The listing builds one solid part. Answer for the finished solid, in the listing's coordinates (mm). A direction names the side the tool comes from. Coordinates: 2 decimals unless noted, no trailing zeros. Order: outer loops, then holes, each group sorted by start corner. A loop starts at its lowest first (then second) coordinate and runs counter-clockwise, first axis right, second up. Notation, with made-up numbers: (-9.5, 78) -> (22.5, 78) arc R24 cw to (22.5, 112) -> close; hole circle Ø11 at (-24.75, 79). An arc over 180 degrees is marked (long way). Return JSON: item names as keys, results as strings.
from build123d import *

# Parameters (mm, degrees)
EXTRUDE_1_DEPTH     = 7
SKETCH_2_R          = 2
CUT_EXTRUDE_1_DEPTH = 10
SKETCH_3_W          = 40
SKETCH_3_H          = 40
CUT_EXTRUDE_2_DEPTH = 7
FILLET_1_R          = 2
FILLET_2_R          = 2
SKETCH_4_R          = 2
CUT_EXTRUDE_3_DEPTH = 90


with BuildPart() as part:
    # 草图1 → 凸台-拉伸1 (new body)
    with BuildSketch(Plane.XY):
        Polygon((0, 0), (220, 0), (224.357787137, -49.809734905), (-4.357787137, -49.809734905), align=None)
    extrude(amount=EXTRUDE_1_DEPTH)

    # 草图2 → 切除-拉伸1 (cut)
    with BuildSketch(Plane(origin=(0, 0, 0), x_dir=(0, 0, 1), z_dir=(-0.9961946980917453, 0.08715574274766177, 0))):
        with Locations(Location((3.5, -6, 0), (0, 0, 270))):
            Circle(SKETCH_2_R)
        with Locations(Location((3.5, -44, 0), (0, 0, 270))):
            Circle(SKETCH_2_R)
    cut_extrude_1 = extrude(amount=-CUT_EXTRUDE_1_DEPTH, mode=Mode.SUBTRACT)

    # 镜向1: 切除-拉伸1 across plane
    add(cut_extrude_1.mirror(Plane(origin=(110, 0, 0), x_dir=(0, 0, 1), z_dir=(1, 0, 0))), mode=Mode.SUBTRACT)

    # 草图3 → 切除-拉伸2 (cut)
    with BuildSketch(Plane(origin=(0, 0, 0), x_dir=(-1, 0, 0), z_dir=(0, 0, -1))):
        with Locations((-185, -25)):
            Rectangle(SKETCH_3_W, SKETCH_3_H)
        with Locations((-135, -25)):
            Rectangle(SKETCH_3_W, SKETCH_3_H)
        with Locations((-35, -25)):
            Rectangle(SKETCH_3_W, SKETCH_3_H)
        with Locations((-85, -25)):
            Rectangle(SKETCH_3_W, SKETCH_3_H)
    extrude(amount=-CUT_EXTRUDE_2_DEPTH, mode=Mode.SUBTRACT)

    # 圆角1
    fillet_1_edges = [part.edges().sort_by_distance(p)[0] for p in [
        (205, -45, 3.5),
        (205, -5, 3.5),
        (165, -5, 3.5),
        (165, -45, 3.5),
        (115, -45, 3.5),
        (155, -45, 3.5),
        (155, -5, 3.5),
        (115, -5, 3.5),
    ]]
    fillet(fillet_1_edges, radius=FILLET_1_R)

    # 圆角2
    fillet_2_edges = [part.edges().sort_by_distance(p)[0] for p in [
        (15, -5, 3.5),
        (15, -45, 3.5),
        (55, -45, 3.5),
        (55, -5, 3.5),
        (65, -45, 3.5),
        (105, -45, 3.5),
        (105, -5, 3.5),
        (65, -5, 3.5),
    ]]
    fillet(fillet_2_edges, radius=FILLET_2_R)

    # 草图4 → 切除-拉伸3 (cut)
    with BuildSketch(Plane(origin=(0, 0, 0), x_dir=(1, 0, 0), z_dir=(0, 1, 0))):
        with Locations(Location((60, -3.5, 0), (0, 0, 270))):
            Circle(SKETCH_4_R)
        with Locations(Location((160, -3.5, 0), (0, 0, 270))):
            Circle(SKETCH_4_R)
    extrude(amount=-CUT_EXTRUDE_3_DEPTH, mode=Mode.SUBTRACT)


solid = part.part
1. The part is cut by section D-D on y = -11.5. Give the vertices of the cut face in (x, z), and give its area (3 significant figures).
Answer block:
{"outline": "(-1.01, 0) -> (15, 0) -> (15, 7) -> (-1.01, 7) -> close; (55, 0) -> (65, 0) -> (65, 7) -> (55, 7) -> close; (105, 0) -> (115, 0) -> (115, 7) -> (105, 7) -> close; (155, 0) -> (165, 0) -> (165, 7) -> (155, 7) -> close; (205, 0) -> (221.01, 0) -> (221.01, 7) -> (205, 7) -> close; hole circle Ø4 at (60, 3.5); hole circle Ø4 at (160, 3.5)", "area": "409 mm2"}
2. The part is cut by section C-C on x = 60. Give the vertices of the cut face in (y, z).
Answer block:
{"outline": "(-49.81, 0) -> (0, 0) -> (0, 1.5) -> (-49.81, 1.5) -> close; (-49.81, 5.5) -> (0, 5.5) -> (0, 7) -> (-49.81, 7) -> close"}
3. The part is cut by section A-A on x = 145.5. Give the vertices of the cut face in (y, z), and give its area (3 significant figures).
Answer block:
{"outline": "(-49.81, 0) -> (-45, 0) -> (-45, 7) -> (-49.81, 7) -> close; (-5, 0) -> (0, 0) -> (0, 7) -> (-5, 7) -> close", "area": "68.7 mm2"}
4. The part is cut by section B-B on y = -38. Give the vertices of the cut face in (x, z).
Answer block:
{"outline": "(-3.32, 0) -> (15, 0) -> (15, 7) -> (-3.32, 7) -> close; (55, 0) -> (65, 0) -> (65, 7) -> (55, 7) -> close; (105, 0) -> (115, 0) -> (115, 7) -> (105, 7) -> close; (155, 0) -> (165, 0) -> (165, 7) -> (155, 7) -> close; (205, 0) -> (223.32, 0) -> (223.32, 7) -> (205, 7) -> close; hole circle Ø4 at (60, 3.5); hole circle Ø4 at (160, 3.5)"}
5. Determine the mould class of faces 4 (the face through (112, -49.81, 3)), 5 (the face through (85, -5, 3)), 6 (the face through (222.15, -24.56, 3.45)) for opening direction X: pulls with the +X half, pulls with the -X half, needs draft (parallel to the pull), parting line crosses it, or undercut.
Answer block:
{"face 4": "needs draft", "face 5": "undercut", "face 6": "pulls with the +X half"}
6. For faces 1 (the face through (9.44, -6.82, 3.53)), 2 (the face through (158.226, -24.556, 4.423)), 3 (the face through (135, -5, 3)), determine the directions among +Z, -Z, +X, -X, +Y, -Y from which every point of the face is accessible in a straight line to the end or side of a thin tool.
Answer block:
{"face 1": "none", "face 2": "+Y, -Y", "face 3": "+Z, -Z"}
7. Each of these flat-tipped pins is pushed along its axis until it touches: pin 1 Ø2 at (x, z) = (185.5, 3.5) entering from +Y; pin 2 Ø3 at (y, z) = (-21, 5.5) entering from +X; pin 3 Ø2 at (y, z) = (-23, 4.5) entering from -X; pin 4 Ø2 at (y, z) = (-17, 3.5) entering from +X. Where does it stop, or does it pass through?
Answer block:
{"pin 1": "stops at y = 0", "pin 2": "stops at x = 221.97", "pin 3": "stops at x = -2.1", "pin 4": "stops at x = 221.57"}
8. Consider line 1 (Y direction, x = 21, z = 2.5); line 2 (Z direction, x = 160, y = -13.5); line 3 (X direction, y = -6, z = 6.25). Determine where each line is inside the solid, lowest interval first. Write a range as from..to.
Answer block:
{"line 1": "y = -49.81..-45, -5..0", "line 2": "z = 0..1.5, 5.5..7", "line 3": "x = -0.52..15.27, 54.73..65.27, 104.73..115.27, 154.73..165.27, 204.73..220.52"}
